Study the drawing (mm; zero at the part's minimum x, y, z) and answer. Round coordinates to 2 decimals unless told otherwise and drop trailing zeros. Order: outer loops, then holes, each group sorted by start corner. A loop starts at its lowest first (then second) coordinate and runs counter-clockwise, first axis right, second up. Notation, with made-up numbers: M 32.25,21.5 L 54.25,21.5 A23 ccw 54.25,42.5 Z; hole C -12.75,50 d8. An arc over 180 degrees is marked long. Put each result on its own line as item: value. Start each with the question number.
1. The part is cut by section A-A (x = 35). Give the vertices of the cut face in (y, z).
2. The part is cut by section B-B (z = 2.5). Give the vertices of the cut face in (x, y).
3. Consider line 1 (Y direction, x = 10, z = 2.5); line 2 (Y direction, x = 35, z = 7); line 3 (Y direction, x = 9, z = 1.5). Determine where each line is inside the solid, lowest interval first.
4. Each of these flat-tipped pins is pushed along its axis until it touches: pin 1 Ø1 at (x, z) = (12, 3) entering from -Y; pin 2 Ø1 at (x, y) = (19, 19.5) entering from +Z. Where does it stop, or does it pass through?
5. The part is cut by section D-D (x = 10). Give the vertices of the cut face in (y, z).
6. The mould has two halves that part along Y. Classify the marked faces 1, 2, 3 and 4: +Y half, -Y half, draft (parallel to the pull), parting line (faces both ways), or undercut.
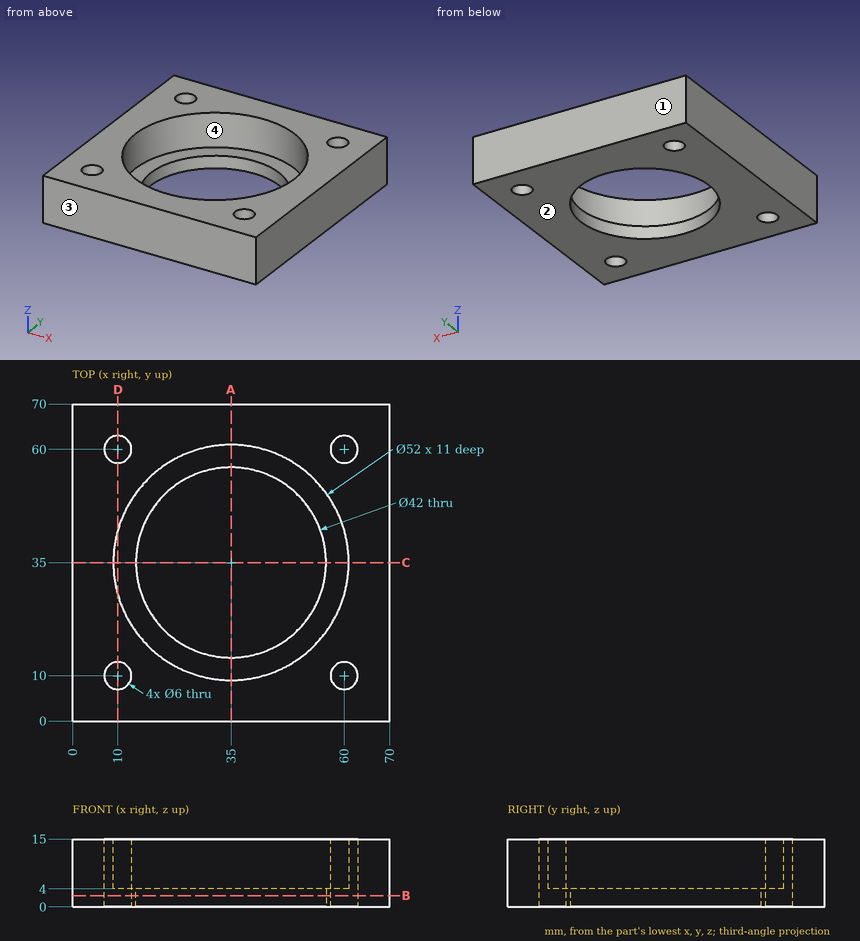
Resolved:
1. outline: M 0,0 L 14,0 L 14,4 L 9,4 L 9,15 L 0,15 Z; M 56,0 L 70,0 L 70,15 L 61,15 L 61,4 L 56,4 Z
2. outline: M 0,0 L 70,0 L 70,70 L 0,70 Z; hole C 10,10 d6; hole C 10,60 d6; hole C 35,35 d42; hole C 60,10 d6; hole C 60,60 d6
3. line 1: 0 to 7, 13 to 57, 63 to 70
3. line 2: 0 to 9, 61 to 70
3. line 3: 0 to 7.17, 12.83 to 57.17, 62.83 to 70
4. pin 1: y = 0
4. pin 2: z = 4
5. outline: M 0,0 L 7,0 L 7,15 L 0,15 Z; M 13,0 L 57,0 L 57,15 L 42.14,15 L 42.14,4 L 27.86,4 L 27.86,15 L 13,15 Z; M 63,0 L 70,0 L 70,15 L 63,15 Z
6. face 1: +Y half
6. face 2: draft
6. face 3: -Y half
6. face 4: undercut
